```python
from build123d import *

# Parameters (mm, degrees)
F1_DEPTH = 609.6
F2_W     = 50.8
F2_H     = 25.4
F3_DEPTH = 609.6
F4_W     = 25.4
F4_H     = 25.4
F5_DEPTH = 609.6
F6_W     = 25.4
F6_H     = 28.575
F7_DEPTH = 609.6
F8_W     = 19.05
F8_H     = 25.4
F8_W_2   = 25.4
F8_H_2   = 38.1
F9_DEPTH = 609.6


with BuildPart() as f1:
    # F0 (on Top) → F1 (new body)
    with BuildSketch(Plane.XY):
        Polygon((0, 609.6), (0, 0), (25.4, 0), (44.45, 0), (44.45, 12.7), (25.4, 12.7), (25.4, 149.225), (44.45, 149.225), (44.45, 161.925), (25.4, 161.925), (25.4, 298.45), (44.45, 298.45), (44.45, 311.15), (25.4, 311.15), (25.4, 447.675), (44.45, 447.675), (44.45, 460.375), (25.4, 460.375), (25.4, 596.9), (44.45, 596.9), (44.45, 609.6), (25.4, 609.6), align=None)
    extrude(amount=F1_DEPTH)

    # F2 (on face) → F3 (join)
    with BuildSketch(Plane.XZ):
        with Locations((25.4, 12.7)):
            Rectangle(F2_W, F2_H)
    extrude(amount=-F3_DEPTH)

    # F4 (on face) → F5 (cut)
    with BuildSketch(Plane.XZ):
        with Locations((12.7, 596.9)):
            Rectangle(F4_W, F4_H)
    extrude(amount=-F5_DEPTH, mode=Mode.SUBTRACT)

    # F6 (on face) → F7 (cut)
    with BuildSketch(Plane.XZ):
        with Locations((38.1, 14.2875)):
            Rectangle(F6_W, F6_H)
    extrude(amount=-F7_DEPTH, mode=Mode.SUBTRACT)

    # F8 (on face) → F9 (join)
    with BuildSketch(Plane.XZ):
        with Locations((34.925, 41.275)):
            Rectangle(F8_W, F8_H)
        with Locations((31.75, 590.55)):
            Rectangle(F8_W_2, F8_H_2)
    extrude(amount=-F9_DEPTH)


solid = f1.part
```
For this review, take the finished solid that the model builds, in its own axes (mm). A direction names the side the tool comes from. Round coordinates to 2 decimals unless told otherwise and drop trailing zeros. Write each loop counter-clockwise with the first axis right and the second up, starting at its lowest first coordinate (ties: lowest second). Pieces come first, ordered by that corner, then holes.
1) Take a section at B-B on z = 67. Give the boundary of the cut face in (x, y) (3 decimals).
Answer below:
outline: (0, 0) - (44.45, 0) - (44.45, 12.7) - (25.4, 12.7) - (25.4, 149.225) - (44.45, 149.225) - (44.45, 161.925) - (25.4, 161.925) - (25.4, 298.45) - (44.45, 298.45) - (44.45, 311.15) - (25.4, 311.15) - (25.4, 447.675) - (44.45, 447.675) - (44.45, 460.375) - (25.4, 460.375) - (25.4, 596.9) - (44.45, 596.9) - (44.45, 609.6) - (0, 609.6) - close
2) Insertion check: pin 1 Ø6 at (x, y) = (35, 178) entering from -Z (3 decimals); pin 2 Ø1 at (y, z) = (170.5, 405.5) entering from +X; pin 3 Ø20.5 at (y, z) = (345, 601.5) entering from -X. Each pin has a flat end and moves straight along its axis. Give the tip position at first contact, or say it passes through.
Answer below:
pin 1: stops at z = 28.575
pin 2: stops at x = 25.4
pin 3: stops at x = 19.05
3) Mouldability with a two-part tool opening along Y and no side actions: class faces 1 (the face through (35, 229, 571.5)), 2 (the face through (35, 378, 53.975)), 3 (the face through (13, 309, 0)) as +Y half, -Y half, draft (parallel to the pull), parting line (faces both ways), or undercut.
Answer below:
face 1: undercut
face 2: undercut
face 3: draft
4) Take a section at A-A on y = 192.5. Give the boundary of the cut face in (x, z) (3 decimals), then the cut area to 3 significant figures.
Answer below:
outline: (0, 0) - (25.4, 0) - (25.4, 28.575) - (44.45, 28.575) - (44.45, 53.975) - (25.4, 53.975) - (25.4, 571.5) - (44.45, 571.5) - (44.45, 609.6) - (19.05, 609.6) - (19.05, 584.2) - (0, 584.2) - close
area: 16,200 mm2
5) Machinability: for faces 4 (the face through (0, 309, 288)), 5 (the face through (9, 301, 584.2)), 6 (the face through (35, 447.675, 309)), which of the approach directions +Z, -Z, +X, -X, +Y, -Y give a long, thin tool a straight path to every point of the face, cutting with its end or side? Answer none if there is none.
Answer below:
face 4: +Z, -Z, -X, +Y, -Y
face 5: +Z, -X, +Y, -Y
face 6: +X
6) For line 1 along Y through (x, z) = (32.5, 432) (3 decimals); line 2 along Z through (x, y) = (42.5, 342.5) (3 decimals); line 3 along Z through (x, y) = (18.5, 204), list the stretches that pass through material, from the lowest coordinate up.
Answer below:
line 1: y = 0 to 12.7, 149.225 to 161.925, 298.45 to 311.15, 447.675 to 460.375, 596.9 to 609.6
line 2: z = 28.575 to 53.975, 571.5 to 609.6
line 3: z = 0 to 584.2
